from build123d import *

# Parameters (mm, degrees)
SKETCH_1_R          = 1.625
EXTRUDE_1_DEPTH     = 3
FILLET_1_R          = 10
SKETCH_3_R          = 1.625
CUT_EXTRUDE_1_DEPTH = 10
CUT_EXTRUDE_2_DEPTH = 10
SKETCH_5_R          = 1.625
CUT_EXTRUDE_3_DEPTH = 10


with BuildPart() as part:
    # Эскиз1 → Бобышка-Вытянуть1 (new body)
    with BuildSketch(Plane.XY):
        with BuildLine():
            ThreePointArc((-32.5, 4), (-35.328427125, -2.828427125), (-28.5, 0))
            Line((-28.5, 0), (28.5, 0))
            ThreePointArc((28.5, 0), (35.328427125, -2.828427125), (32.5, 4))
            Line((32.5, 4), (32.5, 24.5))
            ThreePointArc((32.5, 24.5), (35.328427125, 31.328427125), (28.5, 28.5))
            Line((28.5, 28.5), (-28.5, 28.5))
            ThreePointArc((-28.5, 28.5), (-35.328427125, 31.328427125), (-32.5, 24.5))
            Line((-32.5, 24.5), (-32.5, 4))
        make_face()
        with Locations((-32.5, 0)):
            Circle(SKETCH_1_R, mode=Mode.SUBTRACT)
        with Locations((32.5, 28.5)):
            Circle(SKETCH_1_R, mode=Mode.SUBTRACT)
        with Locations((-32.5, 28.5)):
            Circle(SKETCH_1_R, mode=Mode.SUBTRACT)
        with Locations((32.5, 0)):
            Circle(SKETCH_1_R, mode=Mode.SUBTRACT)
    extrude(amount=EXTRUDE_1_DEPTH)

    # Скругление1
    fillet_1_edges = [part.edges().sort_by_distance(p)[0] for p in [
        (28.5, 0, 1.5),
        (-28.5, 0, 1.5),
        (-32.5, 4, 1.5),
        (-32.5, 24.5, 1.5),
        (-28.5, 28.5, 1.5),
        (28.5, 28.5, 1.5),
        (32.5, 24.5, 1.5),
        (32.5, 4, 1.5),
    ]]
    fillet(fillet_1_edges, radius=FILLET_1_R)

    # Эскиз3 → Вырез-Вытянуть1 (cut)
    with BuildSketch(Plane(origin=(0, 0, 0), x_dir=(-1, 0, 0), z_dir=(0, 0, -1))):
        with Locations((-17.5, 25)):
            Circle(SKETCH_3_R)
        with Locations(Location((17.5, 25, 0), (0, 0, 180))):
            Circle(SKETCH_3_R)
    extrude(amount=-CUT_EXTRUDE_1_DEPTH, mode=Mode.SUBTRACT)

    # Эскиз4 → Вырез-Вытянуть2 (cut)
    # profile 1 of 2: a face of its own
    with BuildSketch(Plane.XY.offset(3)):
        with BuildLine():
            Line((-8.2, 6.15), (-8.2, 13.85))
            ThreePointArc((-8.2, 13.85), (-8.331801948, 14.168198052), (-8.65, 14.3))
            Line((-8.65, 14.3), (-21.15, 14.3))
            ThreePointArc((-21.15, 14.3), (-23.448097039, 13.348097039), (-24.4, 11.05))
            Line((-24.4, 11.05), (-24.4, 8.95))
            ThreePointArc((-24.4, 8.95), (-23.448097039, 6.651902961), (-21.15, 5.7))
            Line((-21.15, 5.7), (-8.65, 5.7))
            ThreePointArc((-8.65, 5.7), (-8.331801948, 5.831801948), (-8.2, 6.15))
        make_face()
        with BuildLine():
            ThreePointArc((-21.15, 14.05), (-23.271320344, 13.171320344), (-24.15, 11.05))
            Line((-24.15, 11.05), (-24.15, 8.95))
            ThreePointArc((-24.15, 8.95), (-23.271320344, 6.828679656), (-21.15, 5.95))
            Line((-21.15, 5.95), (-8.65, 5.95))
            ThreePointArc((-8.65, 5.95), (-8.508578644, 6.008578644), (-8.45, 6.15))
            Line((-8.45, 6.15), (-8.45, 13.85))
            ThreePointArc((-8.45, 13.85), (-8.508578644, 13.991421356), (-8.65, 14.05))
            Line((-8.65, 14.05), (-21.15, 14.05))
        make_face(mode=Mode.SUBTRACT)
    # profile 2 of 2: a face of its own
    with BuildSketch(Plane.XY.offset(3)):
        with BuildLine():
            ThreePointArc((8.65, 5.7), (8.331801948, 5.831801948), (8.2, 6.15))
            Line((8.2, 6.15), (8.2, 13.85))
            ThreePointArc((8.2, 13.85), (8.331801948, 14.168198052), (8.65, 14.3))
            Line((8.65, 14.3), (21.15, 14.3))
            ThreePointArc((21.15, 14.3), (23.448097039, 13.348097039), (24.4, 11.05))
            Line((24.4, 11.05), (24.4, 8.95))
            ThreePointArc((24.4, 8.95), (23.448097039, 6.651902961), (21.15, 5.7))
            Line((21.15, 5.7), (8.65, 5.7))
        make_face()
        with BuildLine():
            Line((8.45, 6.15), (8.45, 13.85))
            ThreePointArc((8.45, 13.85), (8.508578644, 13.991421356), (8.65, 14.05))
            Line((8.65, 14.05), (21.15, 14.05))
            ThreePointArc((21.15, 14.05), (23.271320344, 13.171320344), (24.15, 11.05))
            Line((24.15, 11.05), (24.15, 8.95))
            ThreePointArc((24.15, 8.95), (23.271320344, 6.828679656), (21.15, 5.95))
            Line((21.15, 5.95), (8.65, 5.95))
            ThreePointArc((8.65, 5.95), (8.508578644, 6.008578644), (8.45, 6.15))
        make_face(mode=Mode.SUBTRACT)
    extrude(amount=-CUT_EXTRUDE_2_DEPTH, mode=Mode.SUBTRACT)


with BuildPart() as body_2:
    # of the pieces the cut leaves, the one that is kept (cut_extrude_2_keep)
    add(part.part.solids().sort_by_distance((-32.5, 18.702041029, 0))[0])

    # Эскиз5 → Вырез-Вытянуть3 (cut)
    with BuildSketch(Plane(origin=(0, 0, 0), x_dir=(-1, 0, 0), z_dir=(0, 0, -1))):
        with Locations((26.6, 10)):
            Circle(SKETCH_5_R)
        with Locations((-26.6, 10)):
            Circle(SKETCH_5_R)
        with Locations((-6, 10)):
            Circle(SKETCH_5_R)
        with Locations((6, 10)):
            Circle(SKETCH_5_R)
    extrude(amount=-CUT_EXTRUDE_3_DEPTH, mode=Mode.SUBTRACT)


solid = body_2.part
Work out the finished part from the listing and answer in its coordinate system (mm). A direction names the side the tool comes from. Coordinates: 2 decimals unless noted, no trailing zeros. Loops run counter-clockwise (first coordinate to the right, second up) from the corner with the lowest first, then second, coordinate; pieces in that order, holes last. Notation, with made-up numbers: (-9, 64) -> (21, 64) arc R6 ccw to (21, 71) -> close; hole circle Ø10 at (84, 65). An arc over 180 degrees is marked (long way). Answer as CSV lines item,"result".
1) Flat-ended cylindrical pins translate along their axes: pin 1 (1.7 mm diameter, centred on y = 10, z = 1, fed in from +X); pin 2 (1.5 mm diameter, centred on x = -26, z = 0.5, fed in from -Y); pin 3 (1.5 mm diameter, centred on x = 18.5, z = 1, fed in from +Y). Find the tip coordinate at first contact, or state that the pin passes through.
A:
pin 1,"stops at x = 32.52"
pin 2,"stops at y = -0.86"
pin 3,"stops at y = 28.5"
2) For faces 1 (the face through (26.43, 29.22, 1.52)), 2 (the face through (-1, 15, 3)), 3 (the face through (-8.2, 10, 2)), 4 (the face through (-26.53, -0.76, 1.52)), determine the directions among +Z, -Z, +X, -X, +Y, -Y from which every point of the face is accessible in a straight line to the end or side of a thin tool.
A:
face 1,"+Z, -Z, +Y"
face 2,"+Z, +X, -X, +Y, -Y"
face 3,"+Z, -Z"
face 4,"+Z, -Z, -Y"
3) The part is cut by section C-C (x = 26.5). Give the vertices of the cut face in (y, z), and give its area (3 significant figures).
A:
outline,"(-0.75, 0) -> (8.38, 0) -> (8.38, 3) -> (-0.75, 3) -> close; (11.62, 0) -> (29.25, 0) -> (29.25, 3) -> (11.62, 3) -> close"
area,"80.3 mm²"
4) The part is cut by section D-D (y = 25). Give the vertices of the cut face in (x, z) (3 decimals).
A:
outline,"(-34.732, 0) -> (-19.125, 0) -> (-19.125, 3) -> (-34.732, 3) -> close; (-15.875, 0) -> (15.875, 0) -> (15.875, 3) -> (-15.875, 3) -> close; (19.125, 0) -> (34.732, 0) -> (34.732, 3) -> (19.125, 3) -> close"
5) The part is cut by section B-B (y = 13). Give the vertices of the cut face in (x, z), and give its area (3 significant figures).
A:
outline,"(-32.5, 0) -> (-23.75, 0) -> (-23.75, 3) -> (-32.5, 3) -> close; (-8.2, 0) -> (8.2, 0) -> (8.2, 3) -> (-8.2, 3) -> close; (23.75, 0) -> (32.5, 0) -> (32.5, 3) -> (23.75, 3) -> close"
area,"102 mm²"
6) Straight lines are drawn through the part: probe 1 along Y at (x, z) = (17.5, 2.25) (3 decimals); probe 2 along X at (y, z) = (6.5, 2.1); probe 3 along Y at (x, z) = (15.5, 1.6). For each, find the intervals that lie inside material, in ascending order.
A:
probe 1,"y = 0 to 5.7, 14.3 to 23.375, 26.625 to 28.5"
probe 2,"x = -33.06 to -23.29, -8.2 to 8.2, 23.29 to 33.06"
probe 3,"y = 0 to 5.7, 14.3 to 28.5"
7) For a pull along X with two mould halves and no side action, classify faces 5 (the face through (-15, 5.7, 2)), 6 (the face through (-33.26, 5.97, 1.52)), 7 (the face through (32.5, 14, 1)) as released by +X, released by -X, zero draft, split by the parting line, or undercut.
A:
face 5,"undercut"
face 6,"released by -X"
face 7,"released by +X"
8) The part is cut by section A-A (x = -6). Give the vertices of the cut face in (y, z) (3 decimals).
A:
outline,"(0, 0) -> (8.375, 0) -> (8.375, 3) -> (0, 3) -> close; (11.625, 0) -> (28.5, 0) -> (28.5, 3) -> (11.625, 3) -> close"
